Work out the finished part from the listing and answer in its coordinate system (mm). Face numbers are marked on the shaded views. A direction names the side the tool comes from. Round coordinates to 2 decimals unless told otherwise and drop trailing zeros. Write each loop counter-clockwise with the first axis right and the second up, starting at its lowest first coordinate (ties: lowest second). Pieces come first, ordered by that corner, then holes. Notation, with made-up numbers: M 19.5,16.5 L 57.5,16.5 A15 cw 57.5,21.5 Z; hole C -20.5,-1.5 d6. An arc over 180 degrees is marked long. One line per item, written item: value. Start each with the question number.
Q1. A tool of negligible diameter and unlimited length cuts with its end or side. For the marked faces 1 and 2, from which of +Z, -Z, +X, -X, +Y, -Y can it reach the whole face along a straight path? Write none if from no direction.
Q2. Find section A-A (x = 0). Write down the section's boundary in (y, z).
Q3. Consider probe 1 along Y at (x, z) = (3, 15); probe 2 along Z at (x, y) = (-6, 44). Determine where each line is inside the solid, lowest interval first.
Q4. Find section B-B (z = 16.5). Write down the section's boundary in (x, y), and give its area (3 significant figures).
Q5. Find section D-D (x = 7.5). Write down the section's boundary in (y, z).
Q6. Find section C-C (y = 52). Write down the section's boundary in (x, z).
Q7. Given pin 1 Ø16 at (x, z) = (8.5, 8.5) entering from +Y; pin 2 Ø12 at (x, y) = (22.5, 51.5) entering from +Z, each flat-ended and moving along its own axis, determine where each tip first touches the part or whether it passes through.
Autodesk Inventor part; units mm, degrees
ref_plane "YZ Plane" through (0, 0, 0) normal (1, 0, 0) x (0, 1, 0)
ref_plane "XZ Plane" through (0, 0, 0) normal (0, 1, 0) x (-1, 0, 0)
ref_plane "XY Plane" through (0, 0, 0) normal (0, 0, 1) x (1, 0, 0)
sketch "Sketch1" plane through (0, 0, 0) normal (0, 1, 0) x (-1, 0, 0)
  line L0 (33, -27.5) -> (-33, -27.5)
  line L1 (-33, -27.5) -> (-33, 27.5)
  line L2 (-33, 27.5) -> (33, 27.5)
  line L3 (33, 27.5) -> (33, -27.5)
  line L4 (33, -27.5) -> (-33, 27.5) construction
  line L5 (-33, -27.5) -> (33, 27.5) construction
  point P0 (0, 0)
  dimension "d0" = 66
  dimension "d1" = 55
extrude "Plate1" add sketch "Sketch1" along normal blind 0.7937
sketch "Sketch3" plane through (0, 0.7937, 0) normal (0, 1, 0) x (1, 0, 0)
  line L0 (0, 0) -> (-33, 0)
  line L1 (-33, 0) -> (-33, 27.5)
  line L2 (-33, 27.5) -> (0, 27.5)
  line L3 (0, 27.5) -> (0, 0)
  circle A0 centre (-22, 16) radius 1.5
  circle A1 centre (-22, -16) radius 1.5
  circle A2 centre (22, 16) radius 1.5
  circle A3 centre (22, -16) radius 1.5
  line L4 (-22, 11) -> (-22, 21) construction
  line L5 (-20.5, 11) -> (-20.5, 21)
  line L6 (-23.5, 21) -> (-23.5, 11)
  arc A4 (-23.5, 11) -> (-20.5, 11) centre (-22, 11) ccw
  arc A5 (-20.5, 21) -> (-23.5, 21) centre (-22, 21) ccw
  line L7 (20.5, 11) -> (20.5, 21)
  line L8 (23.5, 21) -> (23.5, 11)
  arc A6 (20.5, 11) -> (23.5, 11) centre (22, 11) ccw
  arc A7 (23.5, 21) -> (20.5, 21) centre (22, 21) ccw
  line L9 (-20.5, -11) -> (-20.5, -21)
  line L10 (-23.5, -21) -> (-23.5, -11)
  arc A8 (-20.5, -11) -> (-23.5, -11) centre (-22, -11) ccw
  arc A9 (-23.5, -21) -> (-20.5, -21) centre (-22, -21) ccw
  arc A10 (20.5, -21) -> (23.5, -21) centre (22, -21) ccw
  line L11 (23.5, -21) -> (23.5, -11)
  line L12 (20.5, -11) -> (20.5, -21)
  arc A11 (23.5, -11) -> (20.5, -11) centre (22, -11) ccw
  line L13 (-23.5, 16) -> (-20.5, 16)
  line L14 (-20.5, 16) -> (-20.5, -16)
  line L15 (-20.5, -16) -> (-23.5, -16)
  line L16 (-23.5, -16) -> (-23.5, 16)
  line L17 (20.5, -16) -> (23.5, -16)
  line L18 (23.5, -16) -> (23.5, 16)
  line L19 (23.5, 16) -> (20.5, 16)
  line L20 (20.5, 16) -> (20.5, -16)
  dimension "d22" = 3
  dimension "d23" = 32
  dimension "d24" = 22
  dimension "d48" = 5
  dimension "d49" = 3
extrude "Cut1" cut sketch "Sketch3" against normal blind 0.7937 contours L14 A8 L16 L0 | L0 L16 A4 L14 | A4 L6 A0 L5 | L9 A1 L10 A8 | L13 A0 | A0 L6 A5 L5 | A0 L13 | L15 A1 | L9 A9 L10 A1 | A1 L15 | L19 A2 | L8 A6 L7 A2 | A2 L7 A7 L8 | A2 L19 | L18 A11 L20 A6 | L11 A3 L12 A11 | L17 A3 | L11 A10 L12 A3 | A3 L17
sketch "Sketch2" plane through (-33, 0, -26.7063) normal (0, 0, -1) x (-1, 0, 0)
  line L0 (-66, 0) -> (0, 0)
  line L1 (0, 0) -> (0, 85)
  line L2 (0, 85) -> (-66, 85)
  line L3 (-66, 85) -> (-66, 0)
edge flange "Flange1" height 70 angle 90 thickness 0.7937 bend radius 0.7937 thickness toward (0, 0, -1) relief tear relief width 0.7937 relief depth 0.3969 edges at (0, 0.7937, -27.5) wall of the first edge with corners at (33, 0, -26.7063) (-33, 0, -26.7063) (-33, 85, -26.7063) (33, 85, -26.7063)
bend "Bend1"
corner "Corner1"
sketch "Sketch4" plane through (33, 85, -27.5) normal (0, 0, -1) x (-1, 0, 0)
  line L0 (0, -83.4125) -> (66, -83.4125)
  line L1 (66, 0) -> (66, -83.4125)
  line L2 (0, 0) -> (66, 0)
  line L3 (33, -54) -> (33, -48) construction
  line L4 (35, -54) -> (35, -48)
  line L5 (31, -48) -> (31, -54)
  arc A0 (31, -54) -> (35, -54) centre (33, -54) ccw
  arc A1 (35, -48) -> (31, -48) centre (33, -48) ccw
  line L6 (33, -83.4125) -> (33, 0)
  line L7 (47.5, -44) -> (47.5, -28.5) construction
  line L8 (49.5, -44) -> (49.5, -28.5)
  line L9 (45.5, -28.5) -> (45.5, -44)
  arc A2 (45.5, -44) -> (49.5, -44) centre (47.5, -44) ccw
  arc A3 (49.5, -28.5) -> (45.5, -28.5) centre (47.5, -28.5) ccw
  line L10 (18.5, -44) -> (18.5, -28.5) construction
  line L11 (16.5, -44) -> (16.5, -28.5)
  line L12 (20.5, -28.5) -> (20.5, -44)
  arc A4 (16.5, -44) -> (20.5, -44) centre (18.5, -44) ccw
  arc A5 (20.5, -28.5) -> (16.5, -28.5) centre (18.5, -28.5) ccw
  line L13 (66, -85) -> (0, -85)
  line L14 (16, -50) -> (50, -50)
  line L15 (50, -50) -> (50, -16)
  line L16 (50, -16) -> (16, -16)
  line L17 (16, -16) -> (16, -50)
  circle A6 centre (16, -16) radius 2
  circle A7 centre (16, -50) radius 2
  circle A8 centre (50, -50) radius 2
  line L18 (33, -16) -> (33, -50)
  line L19 (16, -18) -> (16, -14) construction
  line L20 (18, -18) -> (18, -14)
  line L21 (14, -14) -> (14, -18)
  arc A9 (14, -18) -> (18, -18) centre (16, -18) ccw
  arc A10 (18, -14) -> (14, -14) centre (16, -14) ccw
  line L22 (16, -52) -> (16, -48) construction
  line L23 (18, -52) -> (18, -48)
  line L24 (14, -48) -> (14, -52)
  arc A11 (14, -52) -> (18, -52) centre (16, -52) ccw
  arc A12 (18, -48) -> (14, -48) centre (16, -48) ccw
  line L25 (50, -52) -> (50, -48) construction
  line L26 (52, -52) -> (52, -48)
  line L27 (48, -48) -> (48, -52)
  arc A13 (48, -52) -> (52, -52) centre (50, -52) ccw
  arc A14 (52, -48) -> (48, -48) centre (50, -48) ccw
  point P0 (33, -85)
  point P1 (33, -51)
  point P2 (47.5, -36.25)
  point P3 (18.5, -36.25)
  dimension "d25" = 3
  dimension "d26" = 4
  dimension "d29" = 4
  dimension "d30" = 15.5
  dimension "d31" = 14.5
  dimension "d46" = 48.75
  dimension "d47" = 34
  dimension "d50" = 34
  dimension "d51" = 34
  dimension "d52" = 4
  dimension "d53" = 4
  dimension "d54" = 4
  dimension "d55" = 35
  dimension "d56" = 0
  dimension "d57" = 2
  dimension "d58" = 4
  dimension "d59" = 2
  dimension "d60" = 4
  dimension "d61" = 2
  dimension "d62" = 4
extrude "Cut2" cut sketch "Sketch4" against normal blind 0.7937 contours L6 L14 L4 A0 | A0 L5 L14 L6 | L14 L5 A1 L6 | L6 A1 L4 L14 | A7 L17 L14 | L14 L17 A7 | L23 A11 L24 A7 | A7 L17 A12 L23 | A8 L15 L14 | L27 A14 L15 A8 | L14 L15 A8 | A8 L26 A13 L27 | A6 L17 L16 | L16 L17 A6 | L20 A9 L17 A6 | A6 L21 A10 L20 | A7 L24 A12 L17 | L15 A14 L26 A8 | A6 L17 A9 L21 | A2 L9 A3 L8 | L11 A5 L12 A4
fillet "Corner Round1" radius 0.7937 4 edges at (-33, 0.3969, 27.5) (33, 0.3969, 27.5) (33, 85, -27.1031) (-33, 85, -27.1031)
equation "\"d0\" = subframe_x"
equation "\"d1\" = subframe_y"
equation "\"d22\" = m3_diameter"
equation "\"d23\" = 0.4 * frame_y"
equation "\"d24\" = 0.333333 * subframe_x"
equation "\"d49\" = m3_diameter"
equation "\"d20\" = Thickness"
equation "\"d26\" = m4_diameter"
equation "\"d29\" = m4_diameter"
equation "\"d33\" = Thickness"
equation "\"d3\" = BendReliefWidth"
equation "\"d4\" = BendReliefDepth"
equation "\"d5\" = MinimumRemnant"
equation "\"d6\" = BendRadius"
equation "\"d9\" = BendRadius"
equation "\"d11\" = CornerReliefSize"
equation "\"d12\" = GapSize"
equation "\"d13\" = JacobiRadiusSize"
equation "\"BendRadius\" = Thickness"
equation "\"BendReliefWidth\" = Thickness"
equation "\"BendReliefDepth\" = 0.5 * Thickness"
equation "\"CornerReliefSize\" = 4 * Thickness"
equation "\"MinimumRemnant\" = 2 * Thickness"
equation "\"TransitionRadius\" = BendRadius"
equation "\"JacobiRadiusSize\" = BendRadius"
equation "\"GapSize\" = Thickness"
equation "\"sm_thickness\" = 1.5875"
equation "\"very_thick_acrylic\" = 9.45"
equation "\"thick_acrylic\" = 5.88"
equation "\"thin_acrylic\" = 3.15"
equation "\"clear_acrylic\" = 3.15"
equation "\"wood_thickness\" = 6.72"
equation "\"m3_diameter\" = 3"
equation "\"m3_head\" = 6"
equation "\"m4_diameter\" = 4"
equation "\"m5_diameter\" = 5"
equation "\"m5_head\" = 10.3"
equation "\"brass_insert_drill\" = 4"
equation "\"m5_brass_insert_drill\" = 6.7"
equation "\"m3_press_nut_drill\" = 4.5"
equation "\"m5_press_nut_drill\" = 6.5"
equation "\"laser_body_diameter\" = 12"
equation "\"carrier_y\" = 251"
equation "\"carrier_z\" = 12"
equation "\"visor_x\" = 253.925"
equation "\"visor_y\" = 85.6"
equation "\"window_z\" = 332.225"
equation "\"window_y\" = 93.75"
equation "\"window_overlap\" = 48"
equation "\"acrylic_into_frame\" = 5"
equation "\"door_x\" = 251"
equation "\"door_z\" = 332.225"
equation "\"door_overlap\" = 48"
equation "\"linear_bearing_spacing\" = 198"
equation "\"tray_border\" = 25"
equation "\"bed_z\" = 25"
equation "\"crane_x\" = 223"
equation "\"crane_z2\" = 12"
equation "\"switch_spacing\" = 19"
equation "\"frame_top_z\" = 385"
equation "\"frame_bottom_z\" = 275"
equation "\"frame_total_z\" = 661.5875"
equation "\"frame_face_y\" = 45"
equation "\"frame_foot_z\" = 12"
equation "\"frame_screw_from_center\" = 25"
equation "\"laser_y_offset\" = 19.4"
equation "\"laser_diameter\" = 13"
equation "\"laser_z_offset\" = 55"
equation "\"laser_y\" = 15"
equation "\"laser_z\" = 75"
equation "\"laser_gap\" = 1"
equation "\"subframe_x\" = 66"
equation "\"subframe_y\" = 55"
equation "\"galvo_frame_x\" = 66"
equation "\"galvo_frame_z\" = 85"
equation "\"galvo_frame_y_offset\" = 27.5"
equation "\"drawer_x\" = 191.7875"
equation "\"drawer_y\" = 67.5"
equation "\"drawer_support_from_top\" = 48"
equation "\"drawer_screw_from_center\" = 55"
equation "\"nema17_x\" = 43"
equation "\"d2\" = BendRadius"
equation "\"d44\" = galvo_frame_x"
equation "\"al_thickness\" = 1.5875"
equation "\"rivet_diameter\" = 3.3"
equation "\"bend_factor\" = 2.26205"
equation "\"sm_bend\" = 3.591"
equation "\"al_bend\" = 3.591"
equation "\"frame_x\" = 353.375"
equation "\"carrier_z2\" = 25"
equation "\"carrier_y2\" = 76.825"
equation "\"injection_plastic\" = 3.15"
equation "\"handle_d\" = 4.7625"
equation "\"lmk8uu_shaft\" = 15"
equation "\"al2_bend\" = 3.591"
equation "\"al3_bend\" = 3.591"
equation "\"st2_thickness\" = 1.5875"
equation "\"st3_bend\" = 3.591"
equation "\"al1_bend\" = 1.7955"
equation "\"st2_bend\" = 3.591"
equation "\"st1_thickness\" = 0.79375"
equation "\"st3_thickness\" = 1.5875"
equation "\"al1_thickness\" = 0.79375"
equation "\"st1_bend\" = 1.7955"
equation "\"al3_thickness\" = 1.5875"
equation "\"acme_nut_d\" = 19.1"
equation "\"platform_upper_y\" = 46.625"
equation "\"frame_back_z\" = 498.2125"
equation "\"drawer_reservoir_overlap_x\" = 19.20625"
equation "\"acrylic1_thickness\" = 5.88"
equation "\"laserresin\" = 5"
equation "\"platform_fold_x\" = 25"
equation "\"crane_t\" = 1.5875"
equation "\"reservoir_t\" = 0.79375"
equation "\"platform_crane_gap\" = 0.1"
equation "\"al2_thickness\" = 1.5875"
equation "\"laser_holder_z\" = 75"
equation "\"crane_gap\" = 0.1"
equation "\"drawer_gap\" = 0.1"
equation "\"frame_gap\" = 0.1"
equation "\"acrylic3_thickness\" = 3.15"
equation "\"laser_holder_t\" = 0.79375"
equation "\"frame_back_y\" = 53.2125"
equation "\"foot_z\" = 15"
equation "\"drawer_t\" = 0.79375"
equation "\"frame_back_x\" = 268.2125"
equation "\"frame_back_t\" = 0.79375"
equation "\"frame_front_fold\" = 15"
equation "\"acme_nut_upper_d\" = 12.7"
equation "\"platform_t\" = 1.5875"
equation "\"tray_t\" = 5.88"
equation "\"foot_t\" = 0.79375"
equation "\"frame_front_y\" = 55"
equation "\"reservoir_flap_y\" = 20.79375"
equation "\"handle_hole_d\" = 5.0625"
equation "\"acrylic2_thickness\" = 3.15"
equation "\"drawer_fold\" = 15"
equation "\"handle_spacing\" = 50.8"
properties part number "subframe" material "Aluminum 6061"
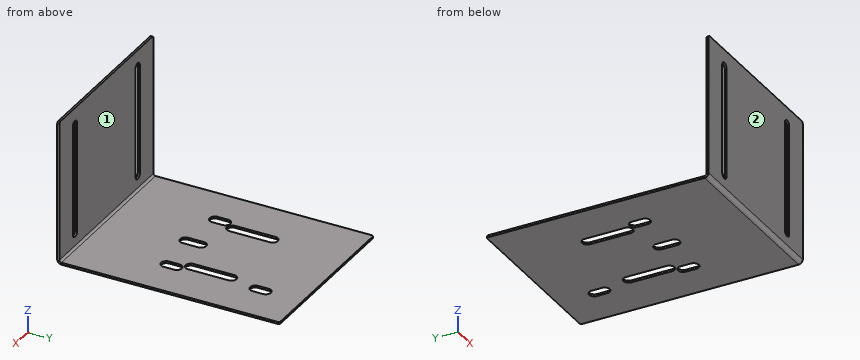
The answers:
1. face 1: +Z, +X, -X, +Y
1. face 2: +Z, -Z, +X, -X, -Y
2. outline: M 0,-25.91 A1.59 ccw 1.59,-27.5 L 29,-27.5 L 29,-26.71 L 1.59,-26.71 A0.79 cw 0.79,-25.91 L 0.79,27.5 L 0,27.5 Z; M 39,-27.5 L 85,-27.5 L 85,-26.71 L 39,-26.71 Z
3. probe 1: 0 to 0.79
3. probe 2: -27.5 to -26.71
4. outline: M -33,0 L -23.5,0 L -23.5,0.79 L -33,0.79 Z; M -20.5,0 L 20.5,0 L 20.5,0.79 L -20.5,0.79 Z; M 23.5,0 L 33,0 L 33,0.79 L 23.5,0.79 Z
4. area: 47.6 mm2
5. outline: M 0,-25.91 A1.59 ccw 1.59,-27.5 L 85,-27.5 L 85,-26.71 L 1.59,-26.71 A0.79 cw 0.79,-25.91 L 0.79,27.5 L 0,27.5 Z
6. outline: M -33,-27.5 L -16.5,-27.5 L -16.5,-26.71 L -33,-26.71 Z; M -12.5,-27.5 L 12.5,-27.5 L 12.5,-26.71 L -12.5,-26.71 Z; M 16.5,-27.5 L 33,-27.5 L 33,-26.71 L 16.5,-26.71 Z
7. pin 1: y = 0.79
7. pin 2: z = -26.71
